Build history of the part. All positions in model axes, mm. Give positions to 0.01 mm unless a question says otherwise; leave off trailing zeros. Order: outer loops, then holes, each group sorted by start corner. A loop starts at its lowest first (then second) coordinate and runs counter-clockwise, first axis right, second up. Notation, with made-up numbers: (12, -5) - (41, -5) arc R14 cw to (41, 17) - close; hole circle Ø4 at (38, 69.25). An arc over 180 degrees is marked (long way). Write each question's results on one line, items separated by ' | '. Start each with the question number.
1) Cut at C-C on x = -19.05. List the corners of the cut face in (y, z) (1 decimal).
2) Cut at B-B on x = 0. List the corners of the cut face in (y, z) (3 decimals), plus the area to 3 significant figures.
3) Cut at D-D on z = -30.5. List the corners of the cut face in (x, y) (3 decimals), plus the area to 3 significant figures.
4) Drill centre lines: line 1 along X through (y, z) = (7.5, -177.8); line 2 along X through (y, z) = (3.5, -177); line 3 along Z through (x, y) = (-19.05, 5.5). Where is each one in solid material? Low to high. Write a range as from..to.
5) Cut at A-A on z = -177.8. List the corners of the cut face in (x, y) (3 decimals), plus the area to 3 significant figures.
6) Drop flat-ended pins along their axis: pin 1 Ø5 at (x, z) = (19.05, -54.991) entering from +Y; pin 2 Ø3 at (y, z) = (3, -23.5) entering from -X; pin 3 Ø5 at (x, y) = (-11.5, 4) entering from -Z; pin 4 Ø13 at (x, z) = (-19.05, -16.891) entering from +Y (3 decimals). Give the stop position or say it passes through.
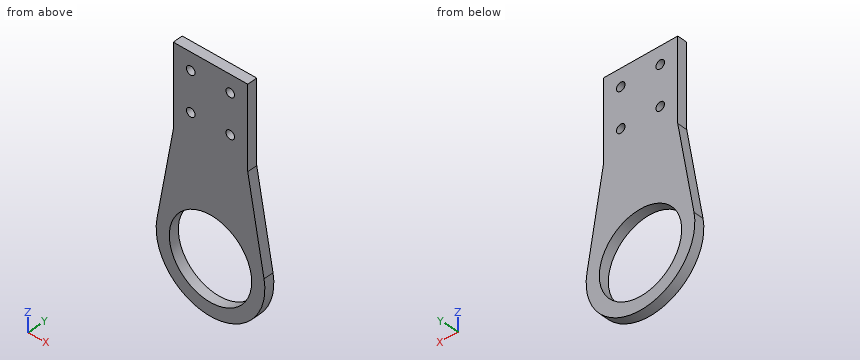
from build123d import *

# Parameters (mm, degrees)
SKETCH1_R           = 39.751
SKETCH1_R_2         = 4.1275
BOSS_EXTRUDE1_DEPTH = 9.525


with BuildPart() as part:
    # Sketch1 → Boss-Extrude1 (new body)
    with BuildSketch(Plane(origin=(0, 0, 0), x_dir=(1, 0, 0), z_dir=(0, 1, 0))):
        with BuildLine():
            Line((-35.941, 0), (35.941, 0))
            Line((35.941, 0), (35.941, 79.578269268))
            Line((35.941, 79.578269268), (51.654151453, 168.691979433))
            ThreePointArc((51.654151453, 168.691979433), (0, 230.251), (-51.654151453, 168.691979433))
            Line((-51.654151453, 168.691979433), (-35.941, 79.578269268))
            Line((-35.941, 79.578269268), (-35.941, 0))
        make_face()
        with Locations((0, 177.8)):
            Circle(SKETCH1_R, mode=Mode.SUBTRACT)
        with Locations((-19.05, 54.991)):
            Circle(SKETCH1_R_2, mode=Mode.SUBTRACT)
        with Locations((19.05, 54.991)):
            Circle(SKETCH1_R_2, mode=Mode.SUBTRACT)
        with Locations((19.05, 16.891)):
            Circle(SKETCH1_R_2, mode=Mode.SUBTRACT)
        with Locations((-19.05, 16.891)):
            Circle(SKETCH1_R_2, mode=Mode.SUBTRACT)
    extrude(amount=BOSS_EXTRUDE1_DEPTH)


solid = part.part
Results:
1) outline: (0, -226.7) - (9.5, -226.7) - (9.5, -212.7) - (0, -212.7) - close; (0, -142.9) - (9.5, -142.9) - (9.5, -59.1) - (0, -59.1) - close; (0, -50.9) - (9.5, -50.9) - (9.5, -21) - (0, -21) - close; (0, -12.8) - (9.5, -12.8) - (9.5, 0) - (0, 0) - close
2) outline: (0, -230.251) - (9.525, -230.251) - (9.525, -217.551) - (0, -217.551) - close; (0, -138.049) - (9.525, -138.049) - (9.525, 0) - (0, 0) - close | area: 1,440 mm^2
3) outline: (-35.941, 0) - (35.941, 0) - (35.941, 9.525) - (-35.941, 9.525) - close | area: 685 mm^2
4) line 1: -52.45..-39.75, 39.75..52.45 | line 2: -52.44..-39.74, 39.74..52.44 | line 3: -226.67..-212.69, -142.91..-59.12, -50.86..-21.02, -12.76..0
5) outline: (-52.451, 0) - (-39.751, 0) - (-39.751, 9.525) - (-52.451, 9.525) - close; (39.751, 0) - (52.451, 0) - (52.451, 9.525) - (39.751, 9.525) - close | area: 242 mm^2
6) pin 1: through | pin 2: x = -35.94 | pin 3: z = -229.47 | pin 4: y = 9.525
